Autodesk Inventor part; units mm, degrees
ref_plane "YZ Plane" through (0, 0, 0) normal (1, 0, 0) x (0, 1, 0)
ref_plane "XZ Plane" through (0, 0, 0) normal (0, 1, 0) x (-1, 0, 0)
ref_plane "XY Plane" through (0, 0, 0) normal (0, 0, 1) x (1, 0, 0)
sketch "Sketch1" plane through (0, 0, 0) normal (0, 0, 1) x (1, 0, 0)
  line L0 (0, 0) -> (0, 40)
  line L1 (0, 40) -> (32, 40)
  line L2 (32, 40) -> (32, 42)
  line L3 (73, 67) -> (73, 47)
  line L4 (73, 47) -> (32, 42)
  line L5 (83, 67) -> (83, 45)
  line L6 (83, 45) -> (85, 45)
  line L7 (83, 67) -> (73, 67)
  line L8 (85, 0) -> (0, 0)
  line L9 (85, 45) -> (85, 0)
  dimension "d1" = 40
  dimension "d2" = 32
  dimension "d4" = 10
  dimension "d5" = 2
  dimension "d6" = 20
  dimension "d9" = 22
  dimension "d10" = 2
  dimension "d11" = 85
revolve "Revolution1" add sketch "Sketch1" angle 360 about axis through (85, 0, 0) along (-1, 0, 0)
sketch "Sketch2" plane through (85, 0, 0) normal (1, 0, 0) x (0, 0, -1)
  circle A0 centre (0, 0) radius 30
  dimension "d13" = 60
extrude "Extrusion1" cut sketch "Sketch2" against normal blind 86
sketch "Sketch3" plane through (85, 0, 0) normal (1, 0, 0) x (0, 0, -1)
  circle A0 centre (0, 60.5) radius 4.5
  circle A1 centre (52.8551, -29.5948) radius 4.5
  circle A2 centre (-52.3945, -30.25) radius 4.5
  circle A3 centre (0, 0) radius 47
  circle A4 centre (0, 0) radius 67
  line L0 (58.0237, -33.5) -> (56.2917, -32.5)
  dimension "d17" = 9
  dimension "d16" = 9
  dimension "d18" = 9
  dimension "d23" = 2
sketch "Sketch4" plane through (83, 0, 0) normal (1, 0, 0) x (0, 0, -1)
  point P0 (0, 0)
extrude "Extrusion2" cut sketch "Sketch3" against normal blind 86 contours A0 | A1 | A2
properties part number "parte eixo"
Read the model definition and answer for the solid it produces. Units are mm, in the model's axes. A direction names the side the tool comes from. Coordinates: 2 decimals unless noted, no trailing zeros. Order: outer loops, then holes, each group sorted by start corner. A loop starts at its lowest first (then second) coordinate and runs counter-clockwise, first axis right, second up. Notation, with made-up numbers: (58.5, -7.75) -> (107.5, -7.75) arc R13 cw to (107.5, 1.25) -> close; hole circle Ø6 at (4, 52.5). An arc over 180 degrees is marked (long way). Answer as a JSON object with one key per item and string values.
1) A cutting plane is placed at D-D, the plane x = 55. Determine the outline of the cut face in (y, z).
Model answer:
{"outline": "circle Ø89.61 at (0, 0); hole circle Ø60 at (0, 0)"}
2) Consider line 1 along Y through (x, z) = (17, 0); line 2 along X through (y, z) = (52.5, -7); line 3 along Y through (x, z) = (61.5, 13). Determine where each line is inside the solid, lowest interval first. Write a range as from..to.
Model answer:
{"line 1": "y = -40..-30, 30..40", "line 2": "x = 73..83", "line 3": "y = -43.71..-27.04, 27.04..43.71"}
3) A cutting plane is placed at C-C, the plane x = 78.5. Determine the outline of the cut face in (y, z).
Model answer:
{"outline": "circle Ø134 at (0, 0); hole circle Ø9 at (-30.25, 52.39); hole circle Ø9 at (-29.59, -52.86); hole circle Ø60 at (0, 0); hole circle Ø9 at (60.5, 0)"}
4) A tool of negligible diameter and unlimited length cuts with its end or side. For faces 4 (the face through (83, 14, 44)), 5 (the face through (32, 37.1, 15.4)), 6 (the face through (77.93, -14.524, 65.407)), from which of +Z, -Z, +X, -X, +Y, -Y can it reach the whole face along a straight path? Write none if from no direction.
Model answer:
{"face 4": "+X", "face 5": "-X", "face 6": "+X, -X"}
5) Each of these flat-tipped pins is pushed along its axis until it touches: pin 1 (10.5 mm diameter, centred on y = 60.5, z = 0, fed in from -X); pin 2 (4 mm diameter, centred on x = 49, z = 27, fed in from -Y); pin 3 (3 mm diameter, centred on x = 59.5, y = 5, fed in from -Z). Where does it stop, or does it pass through?
Model answer:
{"pin 1": "stops at x = 73", "pin 2": "stops at y = -36.33", "pin 3": "stops at z = -45.31"}
6) A cutting plane is placed at A-A, the plane y = 0. Determine the outline of the cut face in (x, z), plus the area to 3 significant figures.
Model answer:
{"outline": "(0, -40) -> (32, -40) -> (32, -42) -> (73, -47) -> (73, -67) -> (83, -67) -> (83, -45) -> (85, -45) -> (85, -30) -> (0, -30) -> close; (0, 30) -> (85, 30) -> (85, 45) -> (83, 45) -> (83, 67) -> (73, 67) -> (73, 47) -> (32, 42) -> (32, 40) -> (0, 40) -> close", "area": "2,630 mm²"}
7) The mould has two halves that part along Y. Classify faces 1 (the face through (73, -46, 14)), 2 (the face through (84.014, 20.765, -39.923)), 3 (the face through (78.07, 56.11, 0.98)): released by +Y, released by -Y, zero draft, split by the parting line, or undercut.
Model answer:
{"face 1": "zero draft", "face 2": "split by the parting line", "face 3": "undercut"}
8) A cutting plane is placed at B-B, the plane z = 0. Determine the outline of the cut face in (x, y).
Model answer:
{"outline": "(0, -40) -> (32, -40) -> (32, -42) -> (73, -47) -> (73, -67) -> (83, -67) -> (83, -45) -> (85, -45) -> (85, -30) -> (0, -30) -> close; (0, 30) -> (85, 30) -> (85, 45) -> (83, 45) -> (83, 56) -> (73, 56) -> (73, 47) -> (32, 42) -> (32, 40) -> (0, 40) -> close; (73, 65) -> (83, 65) -> (83, 67) -> (73, 67) -> close"}
